from build123d import *

# Parameters (mm, degrees)
SKETCH1_W          = 2.41
SKETCH1_H          = 1.5
SKETCH1_3_W        = 2.41
SKETCH1_3_H        = 1.5
CUT_REVOLVE1_ANGLE = 45
CIRPATTERN1_COUNT  = 4
CUT_EXTRUDE1_START = -0.4
SKETCH2_R          = 10
CUT_EXTRUDE1_DEPTH = 2


with BuildPart() as part:
    # Sketch1 → Revolve5 (revolve)
    with BuildSketch(Plane.XY, mode=Mode.PRIVATE) as revolve5_sk:
        with Locations((-1.225318738, 36.465082218)):
            Rectangle(SKETCH1_W, SKETCH1_H)
        with BuildLine():
            Line((-2.430318738, 33.985082218), (-1.735040384, 32.910378534))
            ThreePointArc((-1.735040384, 32.910378534), (-1.343438221, 32.058018495), (-1.209241973, 31.129653665))
            Line((-1.209241973, 31.129653665), (-1.209241973, 28.047788417))
            Line((-1.209241973, 28.047788417), (-0.472655293, 26.909233745))
            Line((-0.472655293, 26.909233745), (-0.472655293, 9.778863627))
            ThreePointArc((-0.472655293, 9.778863627), (-1.478108998, 2.901044306), (-4.410318738, -3.401136412))
            ThreePointArc((-4.410318738, -3.401136412), (-5.901404916, -5.134443013), (-6.678030973, -7.284917782))
            Line((-6.678030973, -7.284917782), (-7.010318738, -9.284917782))
            Line((-7.010318738, -9.284917782), (4.589681262, -9.284917782))
            Line((4.589681262, -9.284917782), (4.589681262, 35.715082218))
            Line((4.589681262, 35.715082218), (-0.020318738, 35.715082218))
            Line((-0.020318738, 35.715082218), (-2.430318738, 35.715082218))
            Line((-2.430318738, 35.715082218), (-2.430318738, 33.985082218))
        make_face()
    revolve(revolve5_sk.sketch.rotate(Axis((4.589681262, -9.284917782, 0), (0, 1, 0)), 270), axis=Axis((4.589681262, -9.284917782, 0), (0, 1, 0)))

    # Sketch1_3 → Cut-Revolve1 (revolve, symmetric, cut)
    with BuildSketch(Plane.XY) as cut_revolve1_sk:
        with Locations((-1.225318738, 36.465082218)):
            Rectangle(SKETCH1_3_W, SKETCH1_3_H)
    cut_revolve1 = revolve(axis=Axis((4.589681262, -9.284917782, 0), (0, 1, 0)), revolution_arc=CUT_REVOLVE1_ANGLE / 2, mode=Mode.SUBTRACT)
    cut_revolve1 = cut_revolve1 + revolve(cut_revolve1_sk.sketch, axis=Axis((4.589681262, -9.284917782, 0), (0, -1, 0)), revolution_arc=CUT_REVOLVE1_ANGLE / 2, mode=Mode.SUBTRACT)

    # CirPattern1: Cut-Revolve1 ×4 about axis
    cirpattern1_axis = Axis((4.589681262, -9.284917782, 0), (0, 1, 0))
    for i in range(1, CIRPATTERN1_COUNT):
        add(cut_revolve1.rotate(cirpattern1_axis, i * 360 / CIRPATTERN1_COUNT), mode=Mode.SUBTRACT)

    # Sketch2 → Cut-Extrude1 (cut)
    with BuildSketch(Plane.XZ.offset(9.284917782).offset(CUT_EXTRUDE1_START)):
        with Locations(Location((4.589681262, 0, 0), (0, 0, 270))):
            Circle(SKETCH2_R)
    extrude(amount=-CUT_EXTRUDE1_DEPTH, mode=Mode.SUBTRACT)


solid = part.part
Source: CAD feature listing. Evaluate the final solid. Frame: model axes, mm. A direction names the side the tool comes from. Round coordinates to 2 decimals unless told otherwise and drop trailing zeros. Order: outer loops, then holes, each group sorted by start corner. A loop starts at its lowest first (then second) coordinate and runs counter-clockwise, first axis right, second up. Notation, with made-up numbers: (31.25, -39) - (58.25, -39) arc R30 ccw to (58.25, -10) - close; hole circle Ø3 at (-32, 13.5). An arc over 180 degrees is marked (long way). Use a Markdown table: item, result. Add a question column.
1. Section query B-B (y = 3). Return the cut outline in (x, z).
2. Set-up query: faces 1 (the cylindrical face through (7.87, 36.48, -3.24)), 2 (the flat face through (2.358, 36.476, 5.388)), 3 (the flat face through (9.978, 36.476, 2.232)), 4 (the flat face through (-0.798, 36.476, -2.232)). Return all of +Z, -Z, +X, -X, +Y, -Y with unobstructed straight access to the full face (end or side cutting, diameter ignored); none if empty.
3. Section query A-A (y = 22). Return the cut outline in (x, z).
4. Mould query, pull axis Y, two halves, no side actions, for faces 5 (the cylindrical face through (-1.16, 29.57, 0.75)), 6 (the flat face through (0, 37.215, 4)), 7 (the flat face through (9.978, 36.476, -2.232)). Classes: +Y half, -Y half, draft (parallel to the pull), parting line (faces both ways), or undercut.
5. Line query: probe 1 along X at (y, z) = (-7.35, 0); probe 2 along Y at (x, z) = (9, 4.5); probe 3 along Y at (x, z) = (11.25, -2). Output: solid intervals per line, ascending.
6. First-contact query: pin 1 (12 mm diameter, centred on x = -1.5, y = 18.5, fed in from +Z); pin 2 (12 mm diameter, centred on x = -4.5, y = 24.5, fed in from +Z); pin 3 (10 mm diameter, centred on y = 26, z = -1.5, fed in from +X). Flat tips, straight axial feed; report the tip coordinate or a pass-through.
Derived:
| question | item | result |
|---|---|---|
| 1 | outline | circle Ø12.08 at (4.59, 0) |
| 2 | face 1 | +Y |
| 2 | face 2 | +Z, +Y |
| 2 | face 3 | +X, +Y |
| 2 | face 4 | -X, +Y |
| 3 | outline | circle Ø10.12 at (4.59, 0) |
| 4 | face 5 | undercut |
| 4 | face 6 | +Y half |
| 4 | face 7 | draft |
| 5 | probe 1 | -6.69 to -5.41, 14.59 to 15.87 |
| 5 | probe 2 | -9.28 to -8.88, -6.88 to 2.16, 32.87 to 37.22 |
| 5 | probe 3 | -9.28 to -8.88, -6.88 to 0.43, 33.88 to 35.72 |
| 6 | pin 1 | z = 5.06 |
| 6 | pin 2 | z = 4.01 |
| 6 | pin 3 | x = 10.39 |
